Read the model definition and answer for the solid it produces. Units are mm, in the model's axes. A direction names the side the tool comes from. Coordinates: 2 decimals unless noted, no trailing zeros. Write each loop counter-clockwise with the first axis right and the second up, starting at its lowest first coordinate (ties: lowest second). Pieces come first, ordered by that corner, then holes. Notation, with made-up numbers: (-9.75, -17.5) -> (14.25, -17.5) arc R17 ccw to (14.25, 15.5) -> close; hole circle Ø4 at (-28.5, 72). An arc over 180 degrees is marked (long way). Answer as a JSON object with one key per item and string values. Group by question number.
(1) Flat-ended cylindrical pins translate along their axes: P1, Ø1.1, axis at x = -22.1, z = 2.66, coming from the +Y side; P2, Ø12, axis at x = -58.5, z = 0.5, coming from the +Y side; P3, Ø10, axis at x = -28.5, y = 18.5, coming from the -Z side. Find the tip coordinate at first contact, or state that the pin passes through.
(2) Straight lines are drawn through the part: L1, parallel to Z at x = -22, y = 32.75; L2, parallel to Y at x = -15, z = 3; L3, parallel to Z at x = -42.5, y = 14.25. For each, find the intervals that lie inside material, in ascending order.
(3) Find section B-B (x = -54). Give the vertices of the cut face in (y, z), then the cut area to 3 significant figures.
(4) For a pull along X with two mould halves and no side action, classify faces 1 (the face through (-15.479, 16.597, -14.803)), 2 (the face through (-31, 11.667, -2)), 3 (the face through (-9.38, 16.74, -11.89)) as +X half, -X half, draft (parallel to the pull), parting line (faces both ways), or undercut.
(5) Which of the six approach directions +Z, -Z, +X, -X, +Y, -Y give full straight-line access (tool end or side, diameter ignored) to faces 4 (the face through (-29.384, 16.737, -16.131)), 5 (the face through (-13.75, 16.74, -15.55)), 6 (the face through (-25.81, 30.22, -4.37))?
(6) Find section C-C (z = 10). Give the vertices of the cut face in (x, y), then the cut area to 3 significant figures.
(7) Find section A-A (y = 28.75). Count the separate pieces of the cut face and the enclosed holes in it, then the cut area to 3 significant figures.
from build123d import *

# Parameters (mm, degrees)
BOSS_EXTRUDE1_DEPTH = 33.333333333
BOSS_EXTRUDE2_DEPTH = 33.333333333
CIRPATTERN2_COUNT   = 13
CIRPATTERN2_ANGLE   = 170
F_20_0MM_1_D        = 20
SCALE_1_SCALE       = 0.3
CUT_EXTRUDE_1_DEPTH = 5.5
SKETCH_2_R          = 5.75
EXTRUDE_1_DEPTH     = 12
SKETCH_3_R          = 0.9
CUT_EXTRUDE_2_DEPTH = 7


with BuildPart() as part:
    # Sketch1 → Boss-Extrude1 (new body)
    with BuildSketch(Plane(origin=(0, 0, 0), x_dir=(1, 0, 0), z_dir=(0, 1, 0))):
        with BuildLine():
            Line((-150, 18), (-46.647615159, 18))
            ThreePointArc((-46.647615159, 18), (50, 0), (-46.647615159, -18))
            Line((-46.647615159, -18), (-150, -18))
            ThreePointArc((-150, -18), (-168, 0), (-150, 18))
        make_face()
    extrude(amount=BOSS_EXTRUDE1_DEPTH)

    # Sketch2 → Boss-Extrude2 (add)
    with BuildSketch(Plane(origin=(0, 33.333333333, 0), x_dir=(1, 0, 0), z_dir=(0, 1, 0))):
        Polygon((49.877349569, 3.5), (60, 2), (60, -2), (49.877349569, -3.5), (50, 0), align=None)
    boss_extrude2 = extrude(amount=-BOSS_EXTRUDE2_DEPTH)

    # CirPattern2: Boss-Extrude2 ×13 about axis
    cirpattern2_axis = Axis((0, 0, 0), (0, 1, 0))
    for i in range(1, CIRPATTERN2_COUNT):
        add(boss_extrude2.rotate(cirpattern2_axis, i * CIRPATTERN2_ANGLE / (CIRPATTERN2_COUNT - 1)))

    # Ø20.0mm 맞춤핀 구멍1 (through all)
    with Locations(Plane(origin=(0, 33.333333333, 0), x_dir=(1, 0, 0), z_dir=(0, 1, 0))):
        with Locations((-150, 0)):
            Hole(F_20_0MM_1_D / 2)


with BuildPart() as part_1:
    # 축척1: scaled about (-31.576481157, 16.666666667, -1.921113945)
    add(part.part.scale(SCALE_1_SCALE).moved(Location((-22.10353681, 11.666666667, -1.344779761))))

    # 스케치1 → 컷-돌출1 (cut)
    with BuildSketch(Plane(origin=(0, 21.666666667, 0), x_dir=(1, 0, 0), z_dir=(0, 1, 0))):
        with BuildLine():
            Line((-36.097821358, -4.055220239), (-67.10353681, -4.055220239))
            ThreePointArc((-67.10353681, -4.055220239), (-72.50353681, 1.344779761), (-67.10353681, 6.744779761))
            Line((-67.10353681, 6.744779761), (-36.097821358, 6.744779761))
            ThreePointArc((-36.097821358, 6.744779761), (-37.10353681, 1.344779761), (-36.097821358, -4.055220239))
        make_face()
    extrude(amount=-CUT_EXTRUDE_1_DEPTH, mode=Mode.SUBTRACT)

    # 스케치2 → 보스-돌출1 (add)
    with BuildSketch(Plane(origin=(0, 21.666666667, 0), x_dir=(1, 0, 0), z_dir=(0, 1, 0))):
        with Locations(Location((-22.10353681, 1.344779761, 0), (0, 0, 270))):
            Circle(SKETCH_2_R)
    extrude(amount=EXTRUDE_1_DEPTH)

    # 스케치3 → 컷-돌출2 (cut)
    with BuildSketch(Plane(origin=(0, 33.666666667, 0), x_dir=(1, 0, 0), z_dir=(0, 1, 0))):
        with Locations(Location((-22.10353681, -2.655220239, 0), (0, 0, 270))):
            Circle(SKETCH_3_R)
        with Locations(Location((-19.275109685, -1.483647363, 0), (0, 0, 270))):
            Circle(SKETCH_3_R)
        with Locations(Location((-18.10353681, 1.344779761, 0), (0, 0, 270))):
            Circle(SKETCH_3_R)
        with Locations(Location((-24.931963935, -1.483647363, 0), (0, 0, 90))):
            Circle(SKETCH_3_R)
        with Locations(Location((-26.10353681, 1.344779761, 0), (0, 0, 90))):
            Circle(SKETCH_3_R)
        with Locations(Location((-24.931963935, 4.173206886, 0), (0, 0, 270))):
            Circle(SKETCH_3_R)
        with Locations(Location((-22.10353681, 5.344779761, 0), (0, 0, 90))):
            Circle(SKETCH_3_R)
        with Locations(Location((-19.275109685, 4.173206886, 0), (0, 0, 90))):
            Circle(SKETCH_3_R)
    extrude(amount=-CUT_EXTRUDE_2_DEPTH, mode=Mode.SUBTRACT)


solid = part_1.part
Results below:
{
 "1": {"P1": "stops at y = 26.67", "P2": "stops at y = 16.17", "P3": "stops at z = -19.21"},
 "2": {"L1": "z = -7.09 to -6.24, -4.45 to 1.76, 3.55 to 4.4", "L2": "y = 11.67 to 21.67", "L3": "z = -6.74 to 4.06"},
 "3": {"outline": "(11.67, -6.74) -> (16.17, -6.74) -> (16.17, 4.06) -> (11.67, 4.06) -> close", "area": "48.6 mm2"},
 "4": {"face 1": "undercut", "face 2": "draft", "face 3": "+X half"},
 "5": {"face 4": "+Y, -Y", "face 5": "-Z, +Y, -Y", "face 6": "+Y"},
 "6": {"outline": "(-31.92, 11.67) -> (-12.29, 11.67) -> (-12.29, 21.67) -> (-31.92, 21.67) -> close", "area": "196 mm2"},
 "7": {"separate pieces": "1", "enclosed holes": "8", "area": "83.5 mm2"}
}
